The listing builds one solid part. Answer for the finished solid, in the listing's coordinates (mm). A direction names the side the tool comes from. Give positions to 0.01 mm unless a question says otherwise; leave off trailing zeros. Loops run counter-clockwise (first coordinate to the right, second up) from the corner with the lowest first, then second, coordinate; pieces in that order, holes last. Notation, with made-up numbers: (42, 23.25) - (61, 23.25) arc R22 ccw to (61, 42.25) - close; hole circle Ø4 at (68, 48). An arc over 180 degrees is marked (long way). Write each question's results on one line, items separated by ' | '.
from build123d import *

# Parameters (mm, degrees)
F0_R     = 2.5
F0_R_2   = 2.51
F0_R_3   = 3.57
F1_DEPTH = 6
F2_R     = 5
F3_DEPTH = 3


with BuildPart() as f1:
    # F0 (on Top) → F1 (new body)
    with BuildSketch(Plane.XY):
        with BuildLine():
            Line((18.83, 25), (-18.83, 25))
            ThreePointArc((-18.83, 25), (-23.192849, 23.192849), (-25, 18.83))
            Line((-25, 18.83), (-25, -18.83))
            ThreePointArc((-25, -18.83), (-23.192849, -23.192849), (-18.83, -25))
            Line((-18.83, -25), (18.83, -25))
            ThreePointArc((18.83, -25), (23.192849, -23.192849), (25, -18.83))
            Line((25, -18.83), (25, 18.83))
            ThreePointArc((25, 18.83), (23.192849, 23.192849), (18.83, 25))
        make_face()
        with Locations((-15, -15.7)):
            Circle(F0_R, mode=Mode.SUBTRACT)
        with Locations((15, -15.7)):
            Circle(F0_R, mode=Mode.SUBTRACT)
        with Locations((0, -10)):
            Circle(F0_R_2, mode=Mode.SUBTRACT)
        with BuildLine():
            Line((-22.255, -3.35), (-22.255, 3.35))
            ThreePointArc((-22.255, 3.35), (-21.005, 4.6), (-19.755, 3.35))
            Line((-19.755, 3.35), (-19.755, -3.35))
            ThreePointArc((-19.755, -3.35), (-21.005, -4.6), (-22.255, -3.35))
        make_face(mode=Mode.SUBTRACT)
        with Locations((-10, 0)):
            Circle(F0_R_2, mode=Mode.SUBTRACT)
        with Locations((-15, 15.7)):
            Circle(F0_R_3, mode=Mode.SUBTRACT)
        with Locations((10, 0)):
            Circle(F0_R_2, mode=Mode.SUBTRACT)
        with Locations((0, 10)):
            Circle(F0_R_2, mode=Mode.SUBTRACT)
        with BuildLine():
            Line((19.755, -3.35), (19.755, 3.35))
            ThreePointArc((19.755, 3.35), (21.005, 4.6), (22.255, 3.35))
            Line((22.255, 3.35), (22.255, -3.35))
            ThreePointArc((22.255, -3.35), (21.005, -4.6), (19.755, -3.35))
        make_face(mode=Mode.SUBTRACT)
        with Locations((15, 15.7)):
            Circle(F0_R_3, mode=Mode.SUBTRACT)
    extrude(amount=F1_DEPTH)

    # F2 (on face) → F3 (cut)
    with BuildSketch(Plane.XY.offset(6)):
        with Locations((0, 10)):
            Circle(F2_R)
        with Locations((0, -10)):
            Circle(F2_R)
    extrude(amount=-F3_DEPTH, mode=Mode.SUBTRACT)


solid = f1.part
Item 1: A cutting plane is placed at D-D, the plane z = 4.85. Count the separate pieces of the cut face and the enclosed holes in it, plus the area to 3 significant figures.
Values found:
separate pieces: 1 | enclosed holes: 10 | area: 2,110 mm²
Item 2: Find the intervals of material crossed by line 1 along Y through (x, z) = (15, 3.85); line 2 along Y through (x, z) = (0, 5); line 3 along X through (y, z) = (-14, 4.55), in increasing order. Write a range as [from, to].
Values found:
line 1: y = [-25, -18.2], [-13.2, 12.13], [19.27, 25] | line 2: y = [-25, -15], [-5, 5], [15, 25] | line 3: x = [-25, -16.83], [-13.17, -3], [3, 13.17], [16.83, 25]
Item 3: Flat-ended cylindrical pins translate along their axes: P1, Ø6, axis at x = 0, y = 10, coming from the -Z side; P2, Ø6.5, axis at x = 0, y = -10, coming from the +Z side. Find the tip coordinate at first contact, or state that the pin passes through.
Values found:
P1: stops at z = 0 | P2: stops at z = 3
Item 4: For faces 1 (the face through (23.145, -23.241, 2.958)), 2 (the face through (-0.651, 14.957, 4.521)), 3 (the face through (19.755, 0, 3)), determine the directions among +Z, -Z, +X, -X, +Y, -Y from which every point of the face is accessible in a straight line to the end or side of a thin tool.
Values found:
face 1: +Z, -Z, +X, -Y | face 2: +Z | face 3: +Z, -Z
Item 5: A cutting plane is placed at B-B, the plane x = -10. Determine the outline of the cut face in (y, z).
Values found:
outline: (-25, 0) - (-2.51, 0) - (-2.51, 6) - (-25, 6) - close; (2.51, 0) - (25, 0) - (25, 6) - (2.51, 6) - close
Item 6: A cutting plane is placed at A-A, the plane y = 0. Determine the outline of the cut face in (x, z) (3 decimals).
Values found:
outline: (-25, 0) - (-22.255, 0) - (-22.255, 6) - (-25, 6) - close; (-19.755, 0) - (-12.51, 0) - (-12.51, 6) - (-19.755, 6) - close; (-7.49, 0) - (7.49, 0) - (7.49, 6) - (-7.49, 6) - close; (12.51, 0) - (19.755, 0) - (19.755, 6) - (12.51, 6) - close; (22.255, 0) - (25, 0) - (25, 6) - (22.255, 6) - close
Item 7: For a pull along X with two mould halves and no side action, classify faces 4 (the face through (-25, 0, 3)), 5 (the face through (12.5, -15.6, 3)), 6 (the face through (23.241, 23.145, 2.958)), 7 (the face through (-21, 4.6, 3)) as released by +X, released by -X, zero draft, split by the parting line, or undercut.
Values found:
face 4: released by -X | face 5: undercut | face 6: released by +X | face 7: undercut
Item 8: A cutting plane is placed at C-C, the plane y = -15.7. Determine the outline of the cut face in (x, z), plus the area to 3 significant figures.
Values found:
outline: (-25, 0) - (-17.5, 0) - (-17.5, 6) - (-25, 6) - close; (-12.5, 0) - (12.5, 0) - (12.5, 6) - (-12.5, 6) - close; (17.5, 0) - (25, 0) - (25, 6) - (17.5, 6) - close | area: 240 mm²
